```python
from build123d import *

# Parameters (mm, degrees)
SKETCH1_W                 = 85.09
SKETCH1_H                 = 55.88
BOSS_EXTRUDE1_DEPTH       = 2.54
F_4_CLEARANCE_HOLE1_D     = 3.2639
F_4_CLEARANCE_HOLE1_DEPTH = 9.652
F_4_CLEARANCE_HOLE1_TIP   = 0.980574487


with BuildPart() as part:
    # Sketch1 → Boss-Extrude1 (new body)
    with BuildSketch(Plane.XY):
        Rectangle(SKETCH1_W, SKETCH1_H)
    extrude(amount=BOSS_EXTRUDE1_DEPTH)

    # #4 Clearance Hole1
    with Locations(Plane.XY.offset(2.54)):
        with Locations((-38.735, 24.13), (38.735, -24.13), (38.735, 24.13)):
            Hole(F_4_CLEARANCE_HOLE1_D / 2, depth=F_4_CLEARANCE_HOLE1_DEPTH)
            with Locations((0, 0, -(F_4_CLEARANCE_HOLE1_DEPTH + F_4_CLEARANCE_HOLE1_TIP / 2))):  # 118° drill point
                Cone(0, F_4_CLEARANCE_HOLE1_D / 2, F_4_CLEARANCE_HOLE1_TIP, mode=Mode.SUBTRACT)


solid = part.part
```
Geometry: final body of the model. Coordinates: model frame, mm. Give positions to 0.01 mm unless a question says otherwise; leave off trailing zeros. Order: outer loops, then holes, each group sorted by start corner. A loop starts at its lowest first (then second) coordinate and runs counter-clockwise, first axis right, second up. Notation, with made-up numbers: (-14, 76.25) -> (36, 76.25) arc R24 cw to (36, 95.25) -> close; hole circle Ø11 at (60, 81). An arc over 180 degrees is marked (long way). Write each question's results on one line, items separated by ' | '. Start each with the question number.
1) First-contact query: pin 1 (3 mm diameter, centred on x = -38.735, y = 24.13, fed in from -Z) (1 decimal); pin 2 (4 mm diameter, centred on x = 38.735, y = 24.13, fed in from -Z). Flat tips, straight axial feed; report the tip coordinate or a pass-through.
2) Draft query along X for faces 1 (the cylindrical face through (37.18, 24.62, 1.25)), 2 (the cylindrical face through (37.23, -24.76, 1.25)), 3 (the flat face through (-1, -27.94, 1)), 4 (the flat face through (42.545, 0, 1)). Return one class per face: pulls with the +X half, pulls with the -X half, needs draft (parallel to the pull), parting line crosses it, or undercut.
3) Section B-B (y = -24.13). Return loops of the section in (x, z) (3 decimals), then the cut area to 3 significant figures.
4) Section A-A (y = 24.13). Return loops of the section in (x, z) (3 decimals), then the cut area to 3 significant figures.
Calculated:
1) pin 1: through | pin 2: z = 0
2) face 1: undercut | face 2: undercut | face 3: needs draft | face 4: pulls with the +X half
3) outline: (-42.545, 0) -> (37.103, 0) -> (37.103, 2.54) -> (-42.545, 2.54) -> close; (40.367, 0) -> (42.545, 0) -> (42.545, 2.54) -> (40.367, 2.54) -> close | area: 208 mm2
4) outline: (-42.545, 0) -> (-40.367, 0) -> (-40.367, 2.54) -> (-42.545, 2.54) -> close; (-37.103, 0) -> (37.103, 0) -> (37.103, 2.54) -> (-37.103, 2.54) -> close; (40.367, 0) -> (42.545, 0) -> (42.545, 2.54) -> (40.367, 2.54) -> close | area: 200 mm2
